Geometry: final body of the model. Coordinates: model frame, mm. A direction names the side the tool comes from. Give positions to 0.01 mm unless a question says otherwise; leave off trailing zeros. Loops run counter-clockwise (first coordinate to the right, second up) from the corner with the lowest first, then second, coordinate; pieces in that order, holes last. Notation, with made-up numbers: (-11, 75) -> (31, 75) arc R17 cw to (31, 107) -> close; hole circle Ø3 at (16, 7.5). An arc over 180 degrees is marked (long way). Answer in a Markdown table with one row per item. Add a question column.
1) Section query C-C (y = 68). Return the cut outline in (x, z).
2) Section query A-A (y = 2). Return the cut outline in (x, z).
3) First-contact query: P1, Ø3.5, axis at x = -56.78, z = -17.41, coming from the -Y side; P2, Ø0.9, axis at x = 48.5, y = -24.5, coming from the -Z side; P3, Ø5, axis at x = -25.5, y = 63, coming from the -Z side; P4, Ø1.7, axis at x = -70, z = 2.5, coming from the -Y side. Flat tips, straight axial feed; report the tip coordinate or a pass-through.
4) Access query for faces 4 (the flat face through (-148.855, 0.9, 0.3)), 5 (the flat face through (-72.655, 73, -25)), 6 (the flat face through (-161, -22.63, -16)), 7 (the flat face through (-55, 71.161, -25)), 8 (the flat face through (-37.73, 73, -25)). Directions: +Z, -Z, +X, -X, +Y, -Y. A direction counts if a zero-diameter tool reaches every point of the face in a straight line with its end or side. Return the directions, or none.
5) Line query: line 1 (Y direction, x = 47, z = -24.5); line 2 (Z direction, x = -149, y = -4); line 3 (Y direction, x = -68.5, z = -15). Output: solid intervals per line, ascending. Write a range as from..to.
6) Section query B-B (x = -62). Return the cut outline in (y, z), plus the area to 3 significant figures.
7) Draft query along X for faces 1 (the flat face through (38.47, 0.9, 0.3)), 2 (the flat face through (-161, -25.729, -14)), 3 (the flat face through (-174.255, 13.5, 0.3)). Return one class per face: +X half, -X half, draft (parallel to the pull), parting line (faces both ways), or undercut.
```python
from build123d import *

# Parameters (mm, degrees)
BOSS_EXTRUDE1_DEPTH = 3.4798
SKETCH2_W           = 25.4
SKETCH2_H           = 3.0988
BOSS_EXTRUDE2_DEPTH = 31.75
SKETCH3_W           = 25.4
SKETCH3_H           = 3.0988
BOSS_EXTRUDE3_DEPTH = 31.75
SKETCH4_W           = 34.925
SKETCH4_H           = 4.709822999
BOSS_EXTRUDE4_DEPTH = 50.8
SKETCH5_R           = 2.54
CUT_EXTRUDE1_DEPTH  = 209.009244951
SKETCH6_R           = 2.54
CUT_EXTRUDE2_DEPTH  = 209.009244951
SKETCH7_R           = 2.54
CUT_EXTRUDE3_DEPTH  = 209.009244951
SKETCH8_R           = 2.54
CUT_EXTRUDE4_DEPTH  = 50.8
SKETCH9_R           = 2.843025999
CUT_EXTRUDE5_DEPTH  = 209.009244951
SKETCH10_R          = 2.846976016
CUT_EXTRUDE6_DEPTH  = 50.8


with BuildPart() as part:
    # Sketch1 → Boss-Extrude1 (new body)
    with BuildSketch(Plane.XY):
        Polygon((-174.254543657, -25.729136112), (-148.854543657, -25.729136112), (-148.854543657, 43.104656603), (38.470456343, 43.104656603), (38.470456343, -25.729136112), (63.870456343, -25.729136112), (63.870456343, 75.870863888), (-174.254543657, 75.870863888), align=None)
    extrude(amount=BOSS_EXTRUDE1_DEPTH)

    # Sketch2 → Boss-Extrude2 (add)
    with BuildSketch(Plane(origin=(0, 0, 0), x_dir=(-1, 0, 0), z_dir=(0, 0, -1))):
        with Locations((-51.170456343, -24.179736112)):
            Rectangle(SKETCH2_W, SKETCH2_H)
    extrude(amount=BOSS_EXTRUDE2_DEPTH)

    # Sketch3 → Boss-Extrude3 (add)
    with BuildSketch(Plane(origin=(0, 0, 0), x_dir=(-1, 0, 0), z_dir=(0, 0, -1))):
        with Locations((161.554543657, -24.179736112)):
            Rectangle(SKETCH3_W, SKETCH3_H)
    extrude(amount=BOSS_EXTRUDE3_DEPTH)

    # Sketch4 → Boss-Extrude4 (add)
    with BuildSketch(Plane(origin=(0, 0, 0), x_dir=(-1, 0, 0), z_dir=(0, 0, -1))):
        with Locations((55.192043657, 73.515952389)):
            Rectangle(SKETCH4_W, SKETCH4_H)
    extrude(amount=BOSS_EXTRUDE4_DEPTH)

    # Sketch5 → Cut-Extrude1 (cut, through all)
    with BuildSketch(Plane.XZ.offset(25.729136112)):
        with Locations(Location((42.280456343, -15.3939186, 0), (0, 0, 270))):
            Circle(SKETCH5_R)
    extrude(amount=-CUT_EXTRUDE1_DEPTH, mode=Mode.SUBTRACT)

    # Sketch6 → Cut-Extrude2 (cut, through all)
    with BuildSketch(Plane.XZ.offset(25.729136112)):
        with Locations(Location((-170.444543657, -17.137609378, 0), (0, 0, 270))):
            Circle(SKETCH6_R)
    extrude(amount=-CUT_EXTRUDE2_DEPTH, mode=Mode.SUBTRACT)

    # Sketch7 → Cut-Extrude3 (cut, through all)
    with BuildSketch(Plane.XZ.offset(25.729136112)):
        with Locations(Location((-152.664543657, -17.404243817, 0), (0, 0, 270))):
            Circle(SKETCH7_R)
    extrude(amount=-CUT_EXTRUDE3_DEPTH, mode=Mode.SUBTRACT)

    # Sketch8 → Cut-Extrude4 (cut)
    with BuildSketch(Plane(origin=(0, -25.729136112, 0), x_dir=(-1, 0, 0), z_dir=(0, -1, 0))):
        with Locations(Location((-60.060456343, 16.178164824, 0), (0, 0, 90))):
            Circle(SKETCH8_R)
    extrude(amount=-CUT_EXTRUDE4_DEPTH, mode=Mode.SUBTRACT)

    # Sketch9 → Cut-Extrude5 (cut, through all)
    with BuildSketch(Plane(origin=(0, 75.870863888, 0), x_dir=(1, 0, 0), z_dir=(0, 1, 0))):
        with Locations(Location((-56.779543657, 17.413178819, 0), (0, 0, 180))):
            Circle(SKETCH9_R)
    extrude(amount=-CUT_EXTRUDE5_DEPTH, mode=Mode.SUBTRACT)

    # Sketch10 → Cut-Extrude6 (cut)
    with BuildSketch(Plane(origin=(0, 75.870863888, 0), x_dir=(1, 0, 0), z_dir=(0, 1, 0))):
        with Locations(Location((-56.779543657, 31.75, 0), (0, 0, 180))):
            Circle(SKETCH10_R)
    extrude(amount=-CUT_EXTRUDE6_DEPTH, mode=Mode.SUBTRACT)


solid = part.part
```
Evaluation:
| question | item | result |
|---|---|---|
| 1 | outline | (-174.25, 0) -> (63.87, 0) -> (63.87, 3.48) -> (-174.25, 3.48) -> close |
| 2 | outline | (-174.25, 0) -> (-148.85, 0) -> (-148.85, 3.48) -> (-174.25, 3.48) -> close; (38.47, 0) -> (63.87, 0) -> (63.87, 3.48) -> (38.47, 3.48) -> close |
| 3 | P1 | through |
| 3 | P2 | z = -31.75 |
| 3 | P3 | z = 0 |
| 3 | P4 | y = 43.1 |
| 4 | face 4 | +Z, -Z, -Y |
| 4 | face 5 | -Z, -X, +Y, -Y |
| 4 | face 6 | -Z, +X, -X, +Y |
| 4 | face 7 | -Z, +X, -X, -Y |
| 4 | face 8 | -Z, +X, +Y, -Y |
| 5 | line 1 | -25.73..-22.63 |
| 5 | line 2 | 0..3.48 |
| 5 | line 3 | 71.16..75.87 |
| 6 | outline | (43.1, 0) -> (71.16, 0) -> (71.16, -50.8) -> (75.87, -50.8) -> (75.87, 3.48) -> (43.1, 3.48) -> close |
| 6 | area | 353 mm² |
| 7 | face 1 | undercut |
| 7 | face 2 | draft |
| 7 | face 3 | -X half |
